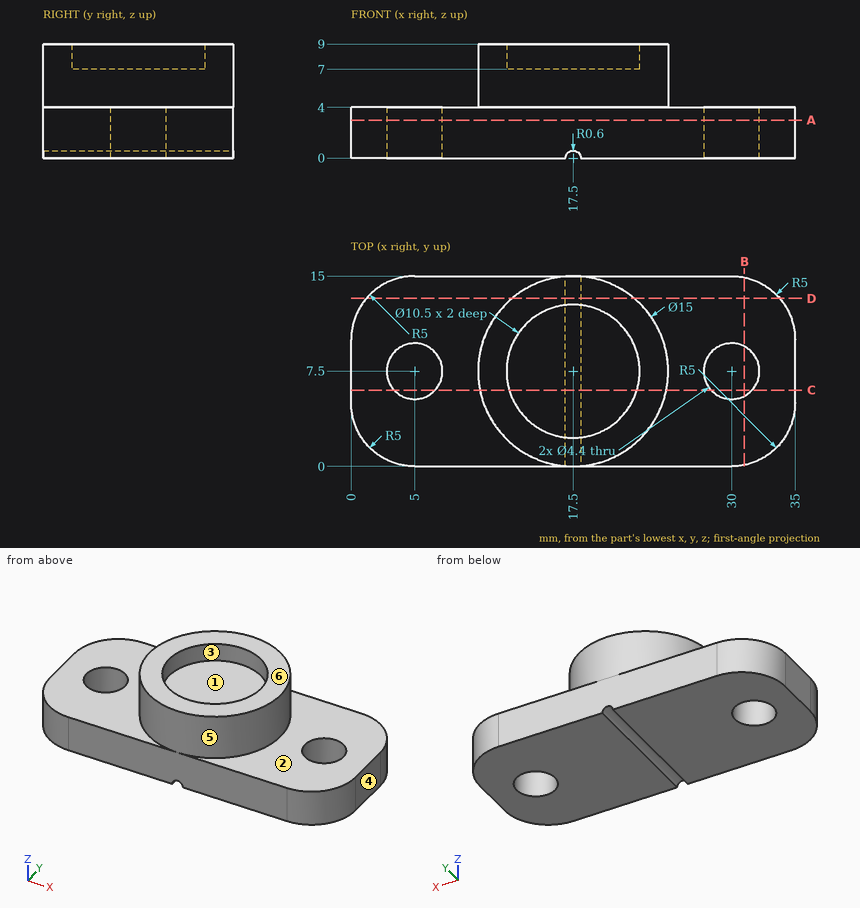
Geometry: see drawing. Coordinates: mm, zero at the bounding-box minimum. A direction names the side the tool comes from. Give positions to 0.01 mm unless a question says otherwise; leave off trailing zeros. Loops run counter-clockwise (first coordinate to the right, second up) from the corner with the lowest first, then second, coordinate; pieces in that order, holes last. Notation, with made-up numbers: (25, 80.25) - (44, 80.25) arc R18 ccw to (44, 84.25) - close; hole circle Ø5 at (38, 70). An arc over 180 degrees is marked (long way). Use CSV: the item, a comma, the result in double quotes. Start each with the question number.
Item 1: Mould query, pull axis X, two halves, no side actions, for the marked faces 1, 2, 3 and 4. Classes: pulls with the +X half, pulls with the -X half, needs draft (parallel to the pull), parting line crosses it, or undercut.
Item 2: Contact query for flat-ended pins moving along their axis: P1, Ø2, axis at x = 4, z = 4.5, coming from the +Y side; P2, Ø1.5, axis at x = 20, y = 5, coming from the +Z side; P3, Ø5, axis at y = 4, z = 5, coming from the -X side; P4, Ø2, axis at y = 13, z = 7.5, coming from the +X side. Output: stop coordinate, or through.
Item 3: Section C-C on y = 6. Return loops of the section in (x, z).
Item 4: Section A-A on z = 3. Return loops of the section in (x, y), then the cut area to 3 significant figures.
Item 5: Reachability of the marked faces 5 and 6 from +Z, -Z, +X, -X, +Y, -Y: full face, straight path, thin tool, end or side. Return the list, or none.
Item 6: Section B-B on x = 31. Return loops of the section in (y, z).
Item 7: Section D-D on y = 13.25. Return loops of the section in (x, z).
Item 8: Line query: line 1 (Y direction, x = 30, z = 2.6); line 2 (Z direction, x = 27, y = 7); line 3 (Z direction, x = 21, y = 8). Output: solid intervals per line, ascending.
Ans:
1,face 1,"undercut"
1,face 2,"needs draft"
1,face 3,"undercut"
1,face 4,"pulls with the +X half"
2,P1,"stops at y = 15"
2,P2,"stops at z = 7"
2,P3,"stops at x = 0"
2,P4,"stops at x = 23.5"
3,outline,"(0, 0) - (3.39, 0) - (3.39, 4) - (0, 4) - close; (6.61, 0) - (16.9, 0) arc R0.6 cw to (18.1, 0) - (28.39, 0) - (28.39, 4) - (24.85, 4) - (24.85, 9) - (22.53, 9) - (22.53, 7) - (12.47, 7) - (12.47, 9) - (10.15, 9) - (10.15, 4) - (6.61, 4) - close; (31.61, 0) - (35, 0) - (35, 4) - (31.61, 4) - close"
4,outline,"(0, 5) arc R5 ccw to (5, 0) - (30, 0) arc R5 ccw to (35, 5) - (35, 10) arc R5 ccw to (30, 15) - (5, 15) arc R5 ccw to (0, 10) - close; hole circle Ø4.4 at (5, 7.5); hole circle Ø4.4 at (30, 7.5)"
4,area,"473 mm2"
5,face 5,"+Z"
5,face 6,"+Z, +X, -X, +Y, -Y"
6,outline,"(0.1, 0) - (5.54, 0) - (5.54, 4) - (0.1, 4) - close; (9.46, 0) - (14.9, 0) - (14.9, 4) - (9.46, 4) - close"
7,outline,"(1.2, 0) - (16.9, 0) arc R0.6 cw to (18.1, 0) - (33.8, 0) - (33.8, 4) - (22.32, 4) - (22.32, 9) - (12.68, 9) - (12.68, 4) - (1.2, 4) - close"
8,line 1,"y = 0 to 5.3, 9.7 to 15"
8,line 2,"z = 0 to 4"
8,line 3,"z = 0 to 7"
